from build123d import *

# Parameters (mm, degrees)
CROQUIS1_R                   = 5.1
SALIENTE_EXTRUIR2_DEPTH      = 2.85
CROQUIS4_R                   = 3.5
SALIENTE_EXTRUIR3_DEPTH      = 2.75
CROQUIS5_R                   = 1.95
SALIENTE_EXTRUIR4_DEPTH      = 3.8
SALIENTE_EXTRUIR5_DEPTH      = 15.2
CORTAR_EXTRUIR4_REACH        = 21.109
CROQUIS8_W                   = 1.085
CROQUIS8_H                   = 2.3
CORTAR_EXTRUIR6_DEPTH        = 10.2
REDONDEO1_R                  = 1
REDONDEO2_R                  = 10
CORTAR_EXTRUIR7_DEPTH        = 0.2
CROQUIS13_R                  = 2.5
CORTAR_EXTRUIR8_DEPTH        = 3.2
CROQUIS14_R                  = 0.9
CORTAR_EXTRUIR9_DEPTH        = 3.7
CORTAR_EXTRUIR10_DEPTH       = 2.65
REDONDEO3_R                  = 0.2
SALIENTE_EXTRUIR6_DEPTH      = 4.55
SALIENTE_EXTRUIR6_DEPTH_BACK = 4.55


with BuildPart() as part:
    # Croquis1 → Saliente-Extruir2 (new body)
    with BuildSketch(Plane(origin=(0, 0, 0), x_dir=(1, 0, 0), z_dir=(0, 1, 0))):
        with Locations(Location((0, 0, 0), (0, 0, 270))):
            Circle(CROQUIS1_R)
    extrude(amount=SALIENTE_EXTRUIR2_DEPTH)

    # Croquis4 → Saliente-Extruir3 (add)
    with BuildSketch(Plane(origin=(0, 2.85, 0), x_dir=(1, 0, 0), z_dir=(0, 1, 0))):
        with Locations(Location((0, 0, 0), (0, 0, 270))):
            Circle(CROQUIS4_R)
    extrude(amount=SALIENTE_EXTRUIR3_DEPTH)

    # Croquis5 → Saliente-Extruir4 (add)
    with BuildSketch(Plane(origin=(0, 5.6, 0), x_dir=(1, 0, 0), z_dir=(0, 1, 0))):
        with Locations(Location((0, 1.55, 0), (0, 0, 89.999128056))):
            Circle(CROQUIS5_R)
    extrude(amount=SALIENTE_EXTRUIR4_DEPTH)

    # Croquis7 → Saliente-Extruir5 (add)
    with BuildSketch(Plane.XY):
        Polygon((0, 2.85), (1.665, 2.85), (1.665, -2.3), (-1.665, -2.3), (-1.665, 2.85), align=None)
    extrude(amount=SALIENTE_EXTRUIR5_DEPTH)

    # Croquis11 → Cortar-Extruir4 (cut, up to next)
    with BuildSketch(Plane(origin=(1.665, 0, 0), x_dir=(0, 0, -1), z_dir=(1, 0, 0)), mode=Mode.PRIVATE) as cortar_extruir4_sk1:
        Polygon((-0.217533037, -2.3), (0, -2.3), (0, 0), (-4.82055754, 0), (-8.216283143, 0), (-12.2, -2.3), align=None)
    cortar_extruir4_tool1 = extrude(cortar_extruir4_sk1.sketch, amount=-CORTAR_EXTRUIR4_REACH, mode=Mode.PRIVATE) & part.part
    add(cortar_extruir4_tool1.solids().sort_by_distance((1.665, -1.224798, 5.168848))[0], mode=Mode.SUBTRACT)

    # Croquis8 → Cortar-Extruir6 (cut)
    with BuildSketch(Plane.XY.offset(15.2)):
        with Locations((-1.1225, -1.15)):
            Rectangle(CROQUIS8_W, CROQUIS8_H)
        with Locations((1.1225, -1.15)):
            Rectangle(CROQUIS8_W, CROQUIS8_H)
    extrude(amount=-CORTAR_EXTRUIR6_DEPTH, mode=Mode.SUBTRACT)

    # Redondeo1
    redondeo1_edges = [part.edges().sort_by_distance(p)[0] for p in [
        (0, -2.3, 12.2),
    ]]
    fillet(redondeo1_edges, radius=REDONDEO1_R)

    # Redondeo2
    redondeo2_edges = [part.edges().sort_by_distance(p)[0] for p in [
        (0, 0, 8.216283143),
    ]]
    fillet(redondeo2_edges, radius=REDONDEO2_R)

    # Croquis12 → Cortar-Extruir7 (cut)
    with BuildSketch(Plane.XZ):
        with BuildLine():
            Line((-0.58, 15.2), (-1.665, 15.2))
            Line((-1.665, 15.2), (-1.665, 4.82055754))
            ThreePointArc((-1.665, 4.82055754), (0, -5.1), (1.665, 4.82055754))
            Line((1.665, 4.82055754), (1.665, 15.2))
            Line((1.665, 15.2), (0.58, 15.2))
            Line((0.58, 15.2), (0.58, 5.536791218))
            Line((0.58, 5.536791218), (0.58, 3.451608321))
            ThreePointArc((0.58, 3.451608321), (0, -3.5), (-0.58, 3.451608321))
            Line((-0.58, 3.451608321), (-0.58, 5.536791218))
            Line((-0.58, 5.536791218), (-0.58, 15.2))
        make_face()
    extrude(amount=-CORTAR_EXTRUIR7_DEPTH, mode=Mode.SUBTRACT)

    # Croquis13 → Cortar-Extruir8 (cut)
    with BuildSketch(Plane.XZ):
        with Locations(Location((0, 0, 0), (0, 0, 270))):
            Circle(CROQUIS13_R)
    extrude(amount=-CORTAR_EXTRUIR8_DEPTH, mode=Mode.SUBTRACT)

    # Croquis14 → Cortar-Extruir9 (cut)
    with BuildSketch(Plane(origin=(0, 9.4, 0), x_dir=(1, 0, 0), z_dir=(0, 1, 0))):
        with Locations(Location((0, 1.55, 0), (0, 0, 270))):
            Circle(CROQUIS14_R)
    extrude(amount=-CORTAR_EXTRUIR9_DEPTH, mode=Mode.SUBTRACT)

    # Croquis15 → Cortar-Extruir10 (cut)
    with BuildSketch(Plane.XZ.offset(-0.2)):
        with BuildLine():
            Line((-4.771792116, 1.8), (-2.999613342, 1.8))
            ThreePointArc((-2.999613342, 1.8), (-3.498239586, 0), (-2.999613342, -1.8))
            Line((-2.999613342, -1.8), (-4.771792116, -1.8))
            ThreePointArc((-4.771792116, -1.8), (-5.1, 0), (-4.771792116, 1.8))
        make_face()
        with BuildLine():
            Line((4.771792116, -1.8), (2.999613342, -1.8))
            ThreePointArc((2.999613342, -1.8), (3.498239586, 0), (2.999613342, 1.8))
            Line((2.999613342, 1.8), (4.771792116, 1.8))
            ThreePointArc((4.771792116, 1.8), (5.1, 0), (4.771792116, -1.8))
        make_face()
    extrude(amount=-CORTAR_EXTRUIR10_DEPTH, mode=Mode.SUBTRACT)

    # Redondeo3
    redondeo3_edges = [part.edges().sort_by_distance(p)[0] for p in [
        (0, -2.3, 15.2),
    ]]
    fillet(redondeo3_edges, radius=REDONDEO3_R)

    # Croquis16 → Saliente-Extruir6 (add, two sides: drawn at the far end of the back side and taken through both)
    with BuildSketch(Plane(origin=(0, 0, 0), x_dir=(0, 0, -1), z_dir=(1, 0, 0)).offset(-SALIENTE_EXTRUIR6_DEPTH_BACK)):
        Polygon((0, 5.6), (1.15, 5.6), (1.15, 4.65), (-1.15, 4.65), (-1.15, 5.6), align=None)
    extrude(amount=SALIENTE_EXTRUIR6_DEPTH + SALIENTE_EXTRUIR6_DEPTH_BACK)


solid = part.part
Part model, mm, in its own coordinate system. A direction names the side the tool comes from. Round coordinates to 2 decimals unless told otherwise and drop trailing zeros. Write each loop counter-clockwise with the first axis right and the second up, starting at its lowest first coordinate (ties: lowest second). Pieces come first, ordered by that corner, then holes. Notation, with made-up numbers: M -28.5,2 L -14.5,2 A19 ccw -14.5,27 Z; hole C 27.5,81 d9. An arc over 180 degrees is marked long. Return JSON: item names as keys, results as strings. Group by question number.
(1) Saw through at D-D on x = 4.25. Write the cut outline in (y, z).
(2) Drill centre lines: probe 1 along X at (y, z) = (1.45, 0); probe 2 along X at (y, z) = (7.75, -1.55); probe 3 along X at (y, z) = (2.5, 8) (3 decimals). Where is each one in solid material? Low to high.
(3) Which spindle directions (+Z, -Z, +X, -X, +Y, -Y) get a long thin tool onto all of the face, cutting with end or side? Do faces 1 (the face through (-0.58, -1, 12)), 2 (the face through (0, 0, 3)), 3 (the face through (4, 5, -1.15)), 4 (the face through (4, 5, 1.15)). Say none if no direction does.
(4) Pin check, flat tips, straight feed: pin 1 Ø1.4 at (x, y) = (3.5, 1.5) entering from -Z; pin 2 Ø1.5 at (y, z) = (2, 8.5) entering from -X (3 decimals); pin 3 Ø0.6 at (x, z) = (-3, -1) entering from -Y; pin 4 Ø2 at (x, z) = (-3, 7) entering from -Y. Stop position of each tip, or through.
(5) Saw through at B-B on x = -4. Write the cut outline in (y, z), then the cut area to 3 significant figures.
(6) Saw through at A-A on y = 0.5. Write the cut outline in (x, z) (3 decimals).
(7) Two-plate mould, pull along X, no slides. Class faces 5 (the face through (-2.44, 1.58, 0.54)), 6 (the face through (0, 3.2, 0)), 7 (the face through (0, 0.2, -4)), 8 (the face through (-3.58, 1.51, 3.63)): +X half, -X half, draft (parallel to the pull), parting line (faces both ways), or undercut.
(8) Saw through at C-C on z = 14.25. Write the cut outline in (x, y) (3 decimals).
Returned:
{
 "1": {"outline": "M 0.2,-2.82 L 2.85,-2.82 L 2.85,-1.8 L 0.2,-1.8 Z; M 0.2,1.8 L 2.85,1.8 L 2.85,2.82 L 0.2,2.82 Z; M 4.65,-1.15 L 5.6,-1.15 L 5.6,1.15 L 4.65,1.15 Z"},
 "2": {"probe 1": "-3.5 to -2.5, 2.5 to 3.5", "probe 2": "-1.95 to -0.9, 0.9 to 1.95", "probe 3": "-1.665 to 1.665"},
 "3": {"face 1": "+Z, -X, -Y", "face 2": "-Z, +X, -X, -Y", "face 3": "-Z, +X, +Y, -Y", "face 4": "+Z, +X, +Y, -Y"},
 "4": {"pin 1": "z = -4.26", "pin 2": "x = -1.665", "pin 3": "y = 0", "pin 4": "through"},
 "5": {"outline": "M 0.2,-3.16 L 2.85,-3.16 L 2.85,-1.8 L 0.2,-1.8 Z; M 0.2,1.8 L 2.85,1.8 L 2.85,3.16 L 0.2,3.16 Z; M 4.65,-1.15 L 5.6,-1.15 L 5.6,1.15 L 4.65,1.15 Z", "area": "9.41 mm²"},
 "6": {"outline": "M -4.772,-1.8 A5.1 ccw 4.772,-1.8 L 3,-1.8 A3.498 ccw 3,1.8 L 4.772,1.8 A5.1 ccw 1.665,4.821 L 1.665,15.2 L -1.665,15.2 L -1.665,4.821 A5.1 ccw -4.772,1.8 L -3,1.8 A3.498 ccw -3,-1.8 Z; hole C 0,0 d5"},
 "7": {"face 5": "undercut", "face 6": "undercut", "face 7": "draft", "face 8": "-X half"},
 "8": {"outline": "M -1.665,0.2 L -0.58,0.2 L -0.58,-2.3 L 0.58,-2.3 L 0.58,0.2 L 1.665,0.2 L 1.665,2.85 L -1.665,2.85 Z"}
}
